Build history of the part. All positions in model axes, mm. A direction names the side the tool comes from. Give positions to 0.01 mm unless a question says otherwise; leave off trailing zeros. Write each loop counter-clockwise with the first axis right and the second up, starting at its lowest first coordinate (ties: lowest second). Pieces come first, ordered by that corner, then holes. Notation, with made-up numbers: (9, 10) -> (40, 10) arc R19 cw to (40, 22) -> close; hole circle Ø11 at (80.5, -16.5). An arc over 180 degrees is marked (long way). Put each result on its own line as item: value.
from build123d import *

# Parameters (mm, degrees)
F0_R     = 31.75
F1_DEPTH = 152.4
F2_W     = 25.4
F2_H     = 12.7


with BuildPart() as f1:
    # F0 (on Front) → F1 (new body)
    with BuildSketch(Plane.XZ):
        Circle(F0_R)
    extrude(amount=-F1_DEPTH)

    # F2 (on Right) → F3 (revolve, cut)
    with BuildSketch(Plane.YZ):
        with Locations((25.4, 25.4)):
            Rectangle(F2_W, F2_H)
    revolve(axis=Axis((0, 76.5412002802, 0), (0, 1, 0)), mode=Mode.SUBTRACT)


solid = f1.part
1) Slice it at C-C (z = 0). Write the cut outline in (x, y).
Filled sheet:
outline: (-31.75, 0) -> (31.75, 0) -> (31.75, 12.7) -> (19.05, 12.7) -> (19.05, 38.1) -> (31.75, 38.1) -> (31.75, 152.4) -> (-31.75, 152.4) -> (-31.75, 38.1) -> (-19.05, 38.1) -> (-19.05, 12.7) -> (-31.75, 12.7) -> close
2) Tool access for faces 5 (the cylindrical face through (29.33, 94.45, -12.16)), 6 (the flat face through (-14, 38.1, -14)): list every direction of +Z, -Z, +X, -X, +Y, -Y with a clear straight run to the whole face (end or side of a thin tool).
Filled sheet:
face 5: +Y, -Y
face 6: none
3) Wall check: L1, parallel to Y at x = -11, z = 23.5; L2, parallel to X at y = 61.5, z = -28; L3, parallel to Z at x = 13, y = 10. Give the ranges that are in metal, low to high.
Filled sheet:
L1: 0 to 12.7, 38.1 to 152.4
L2: -14.97 to 14.97
L3: -28.97 to 28.97
4) Slice it at D-D (y = 26). Write the cut outline in (x, z), plus the area to 3 significant figures.
Filled sheet:
outline: circle Ø38.1 at (0, 0)
area: 1,140 mm2
5) Slice it at B-B (x = 0). Write the cut outline in (y, z), plus the area to 3 significant figures.
Filled sheet:
outline: (0, -31.75) -> (12.7, -31.75) -> (12.7, -19.05) -> (38.1, -19.05) -> (38.1, -31.75) -> (152.4, -31.75) -> (152.4, 31.75) -> (38.1, 31.75) -> (38.1, 19.05) -> (12.7, 19.05) -> (12.7, 31.75) -> (0, 31.75) -> close
area: 9,030 mm2
6) Pin check, flat tips, straight feed: pin 1 (4 mm diameter, centred on x = -6, z = -18, fed in from -Y); pin 2 (12 mm diameter, centred on y = 34.5, z = 10.5, fed in from -X); pin 3 (6 mm diameter, centred on x = -5.5, y = 17.5, fed in from -Z); pin 4 (2 mm diameter, centred on y = 65.5, z = -10.5, fed in from -X). Stop position of each tip, or through.
Filled sheet:
pin 1: y = 0
pin 2: x = -31.23
pin 3: z = -18.89
pin 4: x = -30.3
7) Slice it at A-A (z = -21). Write the cut outline in (x, y).
Filled sheet:
outline: (-23.81, 0) -> (23.81, 0) -> (23.81, 12.7) -> (-23.81, 12.7) -> close; (-23.81, 38.1) -> (23.81, 38.1) -> (23.81, 152.4) -> (-23.81, 152.4) -> close
8) Pull direction Y, two halves, no side cores. Call faces 1 (the cylindrical face through (29.33, 6.26, -12.16)), 2 (the flat face through (-14, 12.7, -14)), 3 (the cylindrical face through (-11.59, 25.58, -15.12)), 4 (the flat face through (0, 152.4, 0)): released by +Y, released by -Y, zero draft, split by the parting line, or undercut.
Filled sheet:
face 1: zero draft
face 2: undercut
face 3: undercut
face 4: released by +Y
